from build123d import *

# Parameters (mm, degrees)
BOSS_EXTRUDE1_DEPTH = 12
BOSS_EXTRUDE2_START = 4
SKETCH2_W           = 10
SKETCH2_H           = 7.500000000000002
SKETCH2_R           = 1.65
BOSS_EXTRUDE2_DEPTH = 4
SKETCH3_W           = 10
SKETCH3_H           = 7.499999999999999
SKETCH3_R           = 1.6500000000000001
BOSS_EXTRUDE3_DEPTH = 4
SKETCH4_R           = 5.000000000000002
BOSS_EXTRUDE4_DEPTH = 25
CUT_EXTRUDE1_DEPTH  = 38.579914848227105
CUT_EXTRUDE2_DEPTH  = 40.44933459514875


with BuildPart() as part:
    # Sketch1 → Boss-Extrude1 (new body)
    with BuildSketch(Plane(origin=(0, 0, 0), x_dir=(1, 0, 0), z_dir=(0, 1, 0))):
        with BuildLine():
            Line((-5, 7.5), (-10, 7.499999999999999))
            Line((-10, 7.499999999999999), (-10, 6.009988028713897))
            ThreePointArc((-10, 6.009988028713897), (-9.937986363684939, 5.515813106068849), (-9.755791145828766, 5.052283767352735))
            Line((-9.755791145828766, 5.052283767352735), (-7.56852494834847, 1.0422957386388614))
            ThreePointArc((-7.56852494834847, 1.042295738638861), (-6.83366266323373, 0.2802022614966764), (-5.812733802519688, -8.9e-16))
            Line((-5.812733802519688, 0), (-5, 0))
            Line((-5, 0), (-5, 2.0999999999999996))
            ThreePointArc((-5.000000000000002, 2.0999999999999996), (-6.65, 3.7500000000000004), (-5, 5.3999999999999995))
            Line((-5, 5.3999999999999995), (-5, 7.5))
        make_face()
        with BuildLine():
            Line((0, 7.5), (-5, 7.5))
            Line((-5, 7.5), (-5, 5.3999999999999995))
            ThreePointArc((-5, 5.3999999999999995), (-3.8332738110421967, 4.916726188957803), (-3.35, 3.7499999999999996))
            ThreePointArc((-3.35, 3.749999999999999), (-3.833273811042198, 2.583273811042195), (-5.000000000000002, 2.0999999999999996))
            Line((-5, 2.0999999999999996), (-5, 0))
            Line((-5, 0), (-4.187266197480313, 0))
            ThreePointArc((-4.187266197480313, -8.9e-16), (-3.1663373367662704, 0.2802022614966755), (-2.4314750516515296, 1.0422957386388605))
            Line((-2.43147505165153, 1.0422957386388614), (-0.24420885417123472, 5.052283767352735))
            ThreePointArc((-0.24420885417123483, 5.052283767352735), (-0.06201363631506229, 5.515813106068849), (0, 6.009988028713897))
            Line((0, 6.009988028713897), (0, 7.5))
        make_face()
    extrude(amount=BOSS_EXTRUDE1_DEPTH)

    # Sketch2 → Boss-Extrude2 (add)
    with BuildSketch(Plane.XZ.offset(BOSS_EXTRUDE2_START)):
        with Locations((-5, -3.75)):
            Rectangle(SKETCH2_W, SKETCH2_H)
        with Locations(Location((-4.999999999999999, -3.75, 0), (0, 0, 270))):
            Circle(SKETCH2_R, mode=Mode.SUBTRACT)
    extrude(amount=-BOSS_EXTRUDE2_DEPTH)

    # Sketch3 → Boss-Extrude3 (add)
    with BuildSketch(Plane(origin=(0, 12, 0), x_dir=(1, 0, 0), z_dir=(0, 1, 0))):
        with Locations((-5, 3.7499999999999996)):
            Rectangle(SKETCH3_W, SKETCH3_H)
        with Locations(Location((-4.999999999999999, 3.7499999999999982, 0), (0, 0, 90))):
            Circle(SKETCH3_R, mode=Mode.SUBTRACT)
    extrude(amount=BOSS_EXTRUDE3_DEPTH)

    # Sketch4 → Boss-Extrude4 (add)
    with BuildSketch(Plane(origin=(-6.5e-16, 0, -7.5), x_dir=(-1, 0, 9e-17), z_dir=(-9e-17, 0, -1))):
        with Locations((5, 6)):
            Circle(SKETCH4_R)
    extrude(amount=BOSS_EXTRUDE4_DEPTH)

    # Sketch5 → Cut-Extrude1 (cut, through all)
    with BuildSketch(Plane(origin=(0, 0, 0), x_dir=(0, 0, -1), z_dir=(1, 0, 0))):
        Polygon((32.5, 11.000000000000002), (7.5, 11), (32.5, 7), align=None)
        Polygon((32.5, 0.9999999999999991), (32.5, 5), (7.5, 0.9999999999999991), align=None)
    extrude(amount=-CUT_EXTRUDE1_DEPTH, mode=Mode.SUBTRACT)

    # Sketch6 → Cut-Extrude2 (cut, through all)
    with BuildSketch(Plane(origin=(0, -4, 0), x_dir=(-1, 0, 0), z_dir=(0, -1, 0))):
        Polygon((3.47e-15, 7.5), (4.000000000000004, 32.50000000000002), (3.92e-15, 32.500000000000014), align=None)
        Polygon((10.000000000000009, 32.500000000000014), (6.000000000000004, 32.500000000000014), (10, 7.5), align=None)
    extrude(amount=-CUT_EXTRUDE2_DEPTH, mode=Mode.SUBTRACT)


solid = part.part
Geometry: final body of the model. Coordinates: model frame, mm. A direction names the side the tool comes from. Round coordinates to 2 decimals unless told otherwise and drop trailing zeros. Loops run counter-clockwise (first coordinate to the right, second up) from the corner with the lowest first, then second, coordinate; pieces in that order, holes last. Notation, with made-up numbers: (51.5, 10) - (106.5, 10) arc R30 ccw to (106.5, 40) - close; hole circle Ø2 at (42, 33). An arc over 180 degrees is marked (long way). Write each question's results on one line, items separated by ' | '. Start each with the question number.
1) Line query: probe 1 along Z at (x, y) = (-5.5, 6.25); probe 2 along X at (y, z) = (10, -3.75); probe 3 along Y at (x, z) = (-6.5, -16). Output: solid intervals per line, ascending. Write a range as [from, to].
2) Cut plane C-C on z = -12.5. Return loops of the section in (x, y).
3) Cut plane A-A on z = -3.75. Return loops of the section in (x, y), then the cut area to 3 significant figures.
4) Mould query, pull axis X, two halves, no side actions, for faces 6 (the face through (-1.45, 2.48, -10.36)), 7 (the face through (-3.39, 5.86, -3.39)), 8 (the face through (-5, 13, -7.5)), 9 (the face through (-8, 6, -20)). Classes: released by +X, released by -X, zero draft, split by the parting line, or undercut.
5) First-contact query: P1, Ø4.5, axis at x = -5, z = -3.75, coming from the -Y side; P2, Ø5, axis at x = -7, z = -18, coming from the +Y side; P3, Ø1.5, axis at x = -6, z = -28.5, coming from the -Y side. Flat tips, straight axial feed; report the tip coordinate or a pass-through.
6) Cut plane D-D on z = -20. Return loops of the section in (x, y), then the cut area to 3 significant figures.
7) Cut plane B-B on z = -27. Return loops of the section in (x, y), then the cut area to 3 significant figures.
8) Access query for faces 1 (the face through (-8.52, 2.45, -10.36)), 2 (the face through (-9, 0, -2)), 3 (the face through (-5, 6, -32.5)), 4 (the face through (0, 5.9, -6.2)), 5 (the face through (-1.353, 5.916, -3.019)). Directions: +Z, -Z, +X, -X, +Y, -Y. A direction counts if a zero-diameter tool reaches every point of the face in a straight line with its end or side. Return the directions, or none.
Verdict:
1) probe 1: z = [-32.5, -5.32], [-2.18, 0] | probe 2: x = [-9.05, -6.65], [-3.35, -0.95] | probe 3: y = [2.36, 9.64]
2) outline: (-9.2, 3.29) arc R5 ccw to (-7.71, 1.8) - (-2.29, 1.8) arc R5 ccw to (-0.8, 3.29) - (-0.8, 8.71) arc R5 ccw to (-2.29, 10.2) - (-7.71, 10.2) arc R5 ccw to (-9.2, 8.71) - close
3) outline: (-10, -4) - (-6.65, -4) - (-6.65, 16) - (-10, 16) - (-10, 12) - (-9.05, 12) - (-9.05, 0) - (-10, 0) - close; (-3.35, -4) - (0, -4) - (0, 0) - (-0.95, 0) - (-0.95, 12) - (0, 12) - (0, 16) - (-3.35, 16) - close | area: 111 mm2
4) face 6: released by +X | face 7: undercut | face 8: zero draft | face 9: released by -X
5) P1: stops at y = -4 | P2: stops at y = 9.72 | P3: stops at y = 4.24
6) outline: (-8, 3) - (-2, 3) - (-2, 9) - (-8, 9) - close | area: 36.0 mm2
7) outline: (-6.88, 4.12) - (-3.12, 4.12) - (-3.12, 7.88) - (-6.88, 7.88) - close | area: 14.1 mm2
8) face 1: -Z, -X, -Y | face 2: +Z, -X | face 3: -Z, +X, -X, +Y, -Y | face 4: +Z, -Z, +X, +Y, -Y | face 5: +Z, +X
